Check sheet for the modelled part. Datum: model origin and axes. Units: mm. Face numbers are marked on the shaded views. A direction names the side the tool comes from. Round coordinates to 2 decimals unless told otherwise and drop trailing zeros. Order: outer loops, then holes, each group sorted by start corner. A loop starts at its lowest first (then second) coordinate and runs counter-clockwise, first axis right, second up.
(1) Thickness scan on probe 1 along X at (y, z) = (10.75, 0); probe 2 along Y at (x, z) = (-5.3, -3.75); probe 3 along Z at (x, y) = (3, 8). Record the ranges inside material, lowest first.
(2) Sectioned sample at B-B, the plane y = 8. Enter the section's corners in (x, z), and give its area (3 significant figures).
(3) Sectioned sample at A-A, the plane x = -5.3. Enter the section's corners in (y, z).
(4) Sectioned sample at C-C, the plane z = -0.5. Enter the section's corners in (x, y), and give its area (3 significant figures).
(5) Sectioned sample at D-D, the plane y = 5.25. Enter the section's corners in (x, z), and give its area (3 significant figures).
(6) Mould release check, pull along X, two halves, no side actions. Record for the marked faces 4, 5 and 6: released by +X, released by -X, zero draft, split by the parting line, or undercut.
(7) Tool access check on the marked faces 1, 2 and 3. Record the directions out of +Z, -Z, +X, -X, +Y, -Y that give a thin tool (end or side, any length) a straight path to the whole face; none if there is none.
(8) Depth check by flat-ended pin: pin 1 (3 mm diameter, centred on x = 5.3, y = 8, fed in from +Z); pin 2 (1.5 mm diameter, centred on x = -5.3, y = 8, fed in from -Z); pin 3 (1.6 mm diameter, centred on y = 7.5, z = -2.5, fed in from -X); pin 4 (5 mm diameter, centred on y = 6.5, z = -1, fed in from -X). Enter the tip coordinate at first touch or a pass-through.
```python
from build123d import *

# Parameters (mm, degrees)
BOSS_EXTRU_1_DEPTH      = 12
ENL_V_MAT_EXTRU_1_REACH = 23.077
ESQUISSE3_R             = 1.25


with BuildPart() as part:
    # Esquisse1 → Boss.-Extru.1 (new body)
    with BuildSketch(Plane(origin=(0, 0, 0), x_dir=(1, 0, 0), z_dir=(0, 1, 0))):
        with BuildLine():
            Line((-10.1, 3.25), (-10.1, -3.25))
            Line((-10.1, -3.25), (-12.1, -3.25))
            Line((-12.1, -3.25), (-15.1, -3.25))
            ThreePointArc((-15.1, -3.25), (-12.978679656, -2.371320344), (-12.1, -0.25))
            Line((-12.1, -0.25), (-12.1, 5.25))
            Line((-12.1, 5.25), (12.1, 5.25))
            Line((12.1, 5.25), (12.1, -0.25))
            ThreePointArc((12.1, -0.25), (12.978679656, -2.371320344), (15.1, -3.25))
            Line((15.1, -3.25), (12.1, -3.25))
            Line((12.1, -3.25), (10.1, -3.25))
            Line((10.1, -3.25), (10.1, 3.25))
            Line((10.1, 3.25), (-10.1, 3.25))
        make_face()
    extrude(amount=BOSS_EXTRU_1_DEPTH)

    # Esquisse3 → Enlèv. mat.-Extru.1 (cut, up to next)
    with BuildSketch(Plane(origin=(0, 0, -5.25), x_dir=(-1, 0, 0), z_dir=(0, 0, -1)), mode=Mode.PRIVATE) as enl_v_mat_extru_1_sk1:
        with Locations((-5.3, 8)):
            Circle(ESQUISSE3_R)
    enl_v_mat_extru_1_tool1 = extrude(enl_v_mat_extru_1_sk1.sketch, amount=-ENL_V_MAT_EXTRU_1_REACH, mode=Mode.PRIVATE) & part.part
    # Esquisse3 → Enlèv. mat.-Extru.1 (cut, up to next)
    with BuildSketch(Plane(origin=(0, 0, -5.25), x_dir=(-1, 0, 0), z_dir=(0, 0, -1)), mode=Mode.PRIVATE) as enl_v_mat_extru_1_sk2:
        with Locations((5.3, 8)):
            Circle(ESQUISSE3_R)
    enl_v_mat_extru_1_tool2 = extrude(enl_v_mat_extru_1_sk2.sketch, amount=-ENL_V_MAT_EXTRU_1_REACH, mode=Mode.PRIVATE) & part.part
    add(enl_v_mat_extru_1_tool1.solids().sort_by_distance((5.3, 8, -5.25))[0], mode=Mode.SUBTRACT)
    add(enl_v_mat_extru_1_tool2.solids().sort_by_distance((-5.3, 8, -5.25))[0], mode=Mode.SUBTRACT)


solid = part.part
```
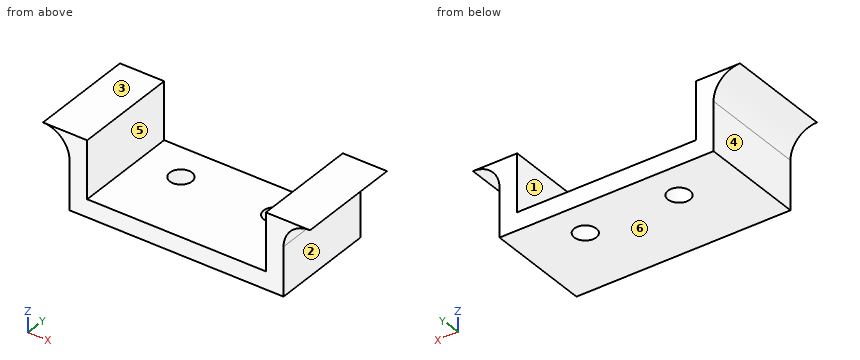
Derived:
1. probe 1: x = -12.1 to -10.1, 10.1 to 12.1
1. probe 2: y = 0 to 6.75, 9.25 to 12
1. probe 3: z = -5.25 to -3.25
2. outline: (-15.1, 3.25) arc R3 cw to (-12.1, 0.25) - (-12.1, -5.25) - (-6.55, -5.25) - (-6.55, -3.25) - (-10.1, -3.25) - (-10.1, 3.25) - close; (-4.05, -5.25) - (4.05, -5.25) - (4.05, -3.25) - (-4.05, -3.25) - close; (6.55, -5.25) - (12.1, -5.25) - (12.1, 0.25) arc R3 cw to (15.1, 3.25) - (10.1, 3.25) - (10.1, -3.25) - (6.55, -3.25) - close
2. area: 68.3 mm2
3. outline: (0, -5.25) - (6.75, -5.25) - (6.75, -3.25) - (0, -3.25) - close; (9.25, -5.25) - (12, -5.25) - (12, -3.25) - (9.25, -3.25) - close
4. outline: (-12.1, 0) - (-10.1, 0) - (-10.1, 12) - (-12.1, 12) - close; (10.1, 0) - (12.1, 0) - (12.1, 12) - (10.1, 12) - close
4. area: 48.0 mm2
5. outline: (-15.1, 3.25) arc R3 cw to (-12.1, 0.25) - (-12.1, -5.25) - (12.1, -5.25) - (12.1, 0.25) arc R3 cw to (15.1, 3.25) - (10.1, 3.25) - (10.1, -3.25) - (-10.1, -3.25) - (-10.1, 3.25) - close
5. area: 78.3 mm2
6. face 4: released by -X
6. face 5: undercut
6. face 6: zero draft
7. face 1: +Z, +Y, -Y
7. face 2: -Z, +X, +Y, -Y
7. face 3: +Z, +X, -X, +Y, -Y
8. pin 1: stops at z = -3.25
8. pin 2: passes through
8. pin 3: stops at x = -12.1
8. pin 4: stops at x = -12.37
